Build history of the part. All positions in model axes, mm. A direction names the side the tool comes from. Round coordinates to 2 decimals unless told otherwise and drop trailing zeros. Loops run counter-clockwise (first coordinate to the right, second up) from the corner with the lowest first, then second, coordinate; pieces in that order, holes last.
from build123d import *

# Parameters (mm, degrees)
F1_DEPTH = 33.02
F2_R     = 3.175
F3_DEPTH = 25.4
F4_R     = 3.175
F5_DEPTH = 25.4


with BuildPart() as f1:
    # F0 (on Front) → F1 (new body)
    with BuildSketch(Plane.XZ):
        Polygon((30.158872, 9.877618), (-20.641128, 9.877618), (-20.641128, 2.257618), (-41.369699, 2.257618), (-41.369699, -2.822382), (-15.969699, -2.822382), (-15.969699, 2.257618), (24.7747, 2.257618), (24.7747, -2.822382), (50.1747, -2.822382), (50.1747, 2.257618), (30.158872, 2.257618), align=None)
    extrude(amount=F1_DEPTH)

    # F2 (on face) → F3 (cut)
    with BuildSketch(Plane.XY.offset(2.257618)):
        with Locations((-31.005413, -28.194)):
            Circle(F2_R)
        with Locations((-31.005413, -4.826)):
            Circle(F2_R)
    extrude(amount=-F3_DEPTH, mode=Mode.SUBTRACT)

    # F4 (on face) → F5 (cut)
    with BuildSketch(Plane.XY.offset(2.257618)):
        with Locations((40.166786, -4.826)):
            Circle(F4_R)
        with Locations((40.166786, -28.194)):
            Circle(F4_R)
    extrude(amount=-F5_DEPTH, mode=Mode.SUBTRACT)


solid = f1.part
(1) Slice it at A-A on x = -31. List the corners of the cut face in (y, z), plus the area to 3 significant figures.
Responses:
outline: (-33.02, -2.82) - (-31.37, -2.82) - (-31.37, 2.26) - (-33.02, 2.26) - close; (-25.02, -2.82) - (-8, -2.82) - (-8, 2.26) - (-25.02, 2.26) - close; (-1.65, -2.82) - (0, -2.82) - (0, 2.26) - (-1.65, 2.26) - close
area: 103 mm2
(2) Probe line 1 (Y direction, x = 40, z = 0); line 2 (X direction, y = -15.5, z = -1.5); line 3 (X direction, y = -27, z = 0). List the from-to ranges inside material, lowest first.
Responses:
line 1: y = -33.02 to -31.36, -25.02 to -8, -1.66 to 0
line 2: x = -41.37 to -15.97, 24.77 to 50.17
line 3: x = -41.37 to -33.95, -28.06 to -15.97, 24.77 to 37.22, 43.11 to 50.17
(3) Which spindle directions (+Z, -Z, +X, -X, +Y, -Y) get a long thin tool onto all of the face, cutting with end or side? Do faces 1 (the face through (-20.641, -16, 6)), 2 (the face through (4, -16, 2.258)), 3 (the face through (41.874, -2.149, -0.247)). Say none if no direction does.
Responses:
face 1: +Z, -X, +Y, -Y
face 2: -Z, +Y, -Y
face 3: +Z, -Z
(4) Pull direction X, two halves, no side cores. Call faces 4 (the face through (30.159, -16, 6)), 5 (the face through (40, -16, 2.258)), 6 (the face through (-27.977, -3.872, -0.247)): +X half, -X half, draft (parallel to the pull), parting line (faces both ways), or undercut.
Responses:
face 4: +X half
face 5: draft
face 6: undercut
(5) Slice it at C-C on y = -11. List the corners of the cut face in (x, z).
Responses:
outline: (-41.37, -2.82) - (-15.97, -2.82) - (-15.97, 2.26) - (24.77, 2.26) - (24.77, -2.82) - (50.17, -2.82) - (50.17, 2.26) - (30.16, 2.26) - (30.16, 9.88) - (-20.64, 9.88) - (-20.64, 2.26) - (-41.37, 2.26) - close
(6) Slice it at D-D on y = -30.5. List the corners of the cut face in (x, z).
Responses:
outline: (-41.37, -2.82) - (-33.19, -2.82) - (-33.19, 2.26) - (-41.37, 2.26) - close; (-28.82, -2.82) - (-15.97, -2.82) - (-15.97, 2.26) - (24.77, 2.26) - (24.77, -2.82) - (37.98, -2.82) - (37.98, 2.26) - (30.16, 2.26) - (30.16, 9.88) - (-20.64, 9.88) - (-20.64, 2.26) - (-28.82, 2.26) - close; (42.35, -2.82) - (50.17, -2.82) - (50.17, 2.26) - (42.35, 2.26) - close
(7) Slice it at B-B on z = -1.5. List the corners of the cut face in (x, y) (3 decimals), plus the area to 3 significant figures.
Responses:
outline: (-41.37, -33.02) - (-15.97, -33.02) - (-15.97, 0) - (-41.37, 0) - close; (24.775, -33.02) - (50.175, -33.02) - (50.175, 0) - (24.775, 0) - close; hole circle Ø6.35 at (-31.005, -28.194); hole circle Ø6.35 at (-31.005, -4.826); hole circle Ø6.35 at (40.167, -28.194); hole circle Ø6.35 at (40.167, -4.826)
area: 1,550 mm2
(8) Pin check, flat tips, straight feed: P1, Ø10.5, axis at x = -27, y = -23, coming from the +Z side; P2, Ø3, axis at x = 21.5, y = -23.5, coming from the -Z side; P3, Ø6, axis at y = -21, z = 6, coming from the +X side. Stop position of each tip, or through.
Responses:
P1: stops at z = 2.26
P2: stops at z = 2.26
P3: stops at x = 30.16
